Autodesk Inventor part; units mm, degrees
ref_plane "YZ Plane" through (0, 0, 0) normal (1, 0, 0) x (0, 1, 0)
ref_plane "XZ Plane" through (0, 0, 0) normal (0, 1, 0) x (-1, 0, 0)
ref_plane "XY Plane" through (0, 0, 0) normal (0, 0, 1) x (1, 0, 0)
sketch "Sketch1" plane through (0, 0, 0) normal (0, 0, 1) x (1, 0, 0)
  line L0 (-750, 0) -> (750, 0) construction
  line L1 (750, 0) -> (750, -2700) construction
  line L2 (750, -2700) -> (-750, -2700) construction
  line L3 (-750, -2700) -> (-750, 0) construction
  line L4 (800, 50) -> (-800, 50) construction
  line L5 (-800, 50) -> (-800, -2750) construction
  line L6 (-800, -2750) -> (800, -2750) construction
  line L7 (800, -2750) -> (800, 50) construction
  line L8 (-850, 100) -> (850, 100) construction
  line L9 (850, 100) -> (850, -2800) construction
  line L10 (850, -2800) -> (-850, -2800) construction
  line L11 (-850, -2800) -> (-850, 100) construction
  arc A0 (750, 0) -> (742.111681, 1.050817) centre (0, -5600) ccw construction
  line L12 (-750, -2100) -> (750, -2100) construction
  line L13 (115.485997, -2697.8227) -> (750, -2100) construction
  arc A1 (750, -2100) -> (750, 0) centre (-10250, -1050) ccw construction
  arc A2 (110, -2700) -> (115.485997, -2697.8227) centre (110, -2692) ccw construction
  arc A3 (742.111681, 1.050817) -> (0, 50) centre (0, -5600) ccw
  line L14 (0, 100) -> (0, 50) construction
  line L15 (0, -2700) -> (0, -2697) construction
  line L16 (0, 47) -> (0, 0) construction
  line L17 (0, 50) -> (0, 47) construction
  line L18 (750.763103, -8.025362) -> (770.411716, -241.9)
  arc A4 (750.763103, -8.025362) -> (742.111681, 1.050817) centre (740.798209, -8.862547) ccw
  point P0 (0, -2750)
  dimension "d54" = 1500
  dimension "d55" = 2700
  dimension "d58" = 2100
  dimension "d83" = 8
  dimension "d113" = 50
  dimension "d114" = 50
  dimension "d115" = 3
  dimension "d121" = 10
  dimension "d122" = 241.9
  dimension "d124" = 94.8023
contour flange "Contour Flange2" sketch "Sketch1" thickness 3 bend radius 5 width 980 along (0, 0, 1) mid plane no both sides no wall seen from (760.58741, -124.962681, 0) lies toward (-0.9964894, -0.0837185, 0) curves L18 A4 A3
bend "Bend2"
corner "Corner2"
mirror "Mirror2" about plane through (0, 0, 0) normal (1, 0, 0)
sketch "Sketch2" plane through (747.773635, -8.276518, 0) normal (-0.9964894, -0.0837185, 0) x (0, 0, 1)
  line L0 (963.847804, -212.844904) -> (852.423188, -212.844904) construction
  line L1 (852.423188, -212.844904) -> (852.423188, -183.740468) construction
  line L2 (852.423188, -183.740468) -> (963.847804, -183.740468) construction
  line L3 (963.847804, -183.740468) -> (963.847804, -212.844904) construction
  point P0 (0, 70.849954)
mark "Mark1"
equation "\"d36\" = Thickness"
equation "\"d37\" = BendReliefWidth"
equation "\"d38\" = BendReliefDepth"
equation "\"d39\" = MinimumRemnant"
equation "\"d40\" = TransitionRadius"
equation "\"d42\" = BendRadius"
equation "\"d44\" = CornerReliefSize"
equation "\"d45\" = GapSize"
equation "\"d46\" = JacobiRadiusSize"
equation "\"BendReliefWidth\" = Thickness"
equation "\"BendReliefDepth\" = 0.5 * Thickness"
equation "\"CornerReliefSize\" = 4 * Thickness"
equation "\"MinimumRemnant\" = 2 * Thickness"
equation "\"GapSize\" = Thickness"
properties part number "MSC 201 SHEET BACK BASIC" material "Stainless Steel AISI 304"
Input: part model. Units: mm. Frame: model coordinates. Coordinates: 2 decimals unless noted, no trailing zeros. Write each loop counter-clockwise with the first axis right and the second up, starting at its lowest first coordinate (ties: lowest second). Pieces come first, ordered by that corner, then holes. Notation, with made-up numbers: (-22.5, -20.5) - (6.5, -20.5) arc R20 cw to (6.5, -11.5) - close; hole circle Ø10 at (-28.5, 32.25). An arc over 180 degrees is marked (long way). Put each result on its own line as item: value. Start each with the question number.
1) Cut plane C-C (x = -279). Return the cut outline in (y, z).
2) Ray query, L1, parallel to X at y = -14, z = 642.5; L2, parallel to X at y = -165, z = 170; L3, parallel to Y at x = -24, z = 539. Return the intervals inside material, ascending.
3) Cut plane A-A (z = 523.5). Return the cut outline in (x, y).
4) Cut plane B-B (y = -218). Return the cut outline in (x, z).
5) Mould query, pull axis X, two halves, no side actions, for faces 1 (the face through (757.46, -123.58, 483.14)), 2 (the face through (-760.725, -126.6, 483.14)), 3 (the face through (-757.735, -126.851, 483.14)), 4 (the face through (760.45, -123.33, 483.14)). Classes: pulls with the +X half, pulls with the -X half, needs draft (parallel to the pull), parting line crosses it, or undercut.
6) Contact query for flat-ended pins moving along their axis: pin 1 (10 mm diameter, centred on y = -191, z = 352, fed in from -X); pin 2 (1.5 mm diameter, centred on y = -85.5, z = 636.5, fed in from -X) (3 decimals); pin 3 (6 mm diameter, centred on y = -3.5, z = 531.5, fed in from -X). Output: stop coordinate, or through.
7) Cut plane D-D (x = 503). Return the cut outline in (y, z), plus the area to 3 significant figures.
Resolved:
1. outline: (40.1, 0) - (43.11, 0) - (43.11, 980) - (40.1, 980) - close
2. L1: x = -751.27 to -748.25, 748.25 to 751.27
2. L2: x = -763.95 to -760.94, 760.94 to 763.95
2. L3: y = 46.95 to 49.95
3. outline: (-770.41, -241.9) - (-767.42, -242.15) - (-747.77, -8.28) arc R7 cw to (-741.72, -1.92) arc R5647 cw to (0, 47) arc R5647 cw to (741.72, -1.92) arc R7 cw to (747.77, -8.28) - (767.42, -242.15) - (770.41, -241.9) - (750.76, -8.03) arc R10 ccw to (742.11, 1.05) arc R5650 ccw to (0, 50) arc R5650 ccw to (-742.11, 1.05) arc R10 ccw to (-750.76, -8.03) - close
4. outline: (-768.4, 0) - (-765.39, 0) - (-765.39, 980) - (-768.4, 980) - close; (765.39, 0) - (768.4, 0) - (768.4, 980) - (765.39, 980) - close
5. face 1: undercut
5. face 2: pulls with the -X half
5. face 3: undercut
5. face 4: pulls with the +X half
6. pin 1: stops at x = -766.56
6. pin 2: stops at x = -757.335
6. pin 3: stops at x = -750.52
7. outline: (24.55, 0) - (27.57, 0) - (27.57, 980) - (24.55, 980) - close
7. area: 2,950 mm2
